Can you work these out from the model? Positions are in its coordinate system, mm. A direction names the side the tool comes from. Coordinates: 2 decimals unless noted, no trailing zeros. Order: outer loops, then holes, each group sorted by start corner. A loop starts at its lowest first (then second) coordinate and runs counter-clockwise, first axis right, second up. Notation, with made-up numbers: M 85.25,-39 L 95.25,-39 A11 cw 95.25,-26 Z; hole C 44.5,-16 d3. An arc over 180 degrees is marked long. Answer as a JSON object with one key per item and string values.
from build123d import *

# Parameters (mm, degrees)
SKETCH1_W                     = 100
SKETCH1_H                     = 100
BOSS_EXTRUDE1_DEPTH           = 2
SKETCH2_W                     = 100
SKETCH2_H                     = 100
SKETCH2_W_2                   = 96
SKETCH2_H_2                   = 96
BOSS_EXTRUDE2_DEPTH           = 30
CHAMFER1_SIZE                 = 10
M3_CLEARANCE_HOLE1_AT_2_COUNT = 2
M3_CLEARANCE_HOLE1_AT_2_PITCH = 10
M3_CLEARANCE_HOLE1_AT_3_COUNT = 2
M3_CLEARANCE_HOLE1_AT_3_PITCH = 19.235384062
M3_CLEARANCE_HOLE1_AT_4_COUNT = 2
M3_CLEARANCE_HOLE1_AT_4_PITCH = 29.154759474
M3_CLEARANCE_HOLE1_AT_5_COUNT = 2
M3_CLEARANCE_HOLE1_AT_5_PITCH = 38.327535793
M3_CLEARANCE_HOLE1_AT_6_COUNT = 2
M3_CLEARANCE_HOLE1_AT_6_PITCH = 48.259714048
CIRPATTERN1_COUNT             = 4


with BuildPart() as part:
    # Sketch1 → Boss-Extrude1 (new body)
    with BuildSketch(Plane(origin=(0, 0, 0), x_dir=(1, 0, 0), z_dir=(0, 1, 0))):
        Rectangle(SKETCH1_W, SKETCH1_H)
    extrude(amount=BOSS_EXTRUDE1_DEPTH)

    # Sketch2 → Boss-Extrude2 (add)
    with BuildSketch(Plane(origin=(0, 2, 0), x_dir=(1, 0, 0), z_dir=(0, 1, 0))):
        Rectangle(SKETCH2_W, SKETCH2_H)
        Rectangle(SKETCH2_W_2, SKETCH2_H_2, mode=Mode.SUBTRACT)
    extrude(amount=BOSS_EXTRUDE2_DEPTH)

    # Chamfer1
    chamfer1_edges = [part.edges().sort_by_distance(p)[0] for p in [
        (-48, 17, -48),
        (-48, 17, 48),
        (48, 17, 48),
        (48, 17, -48),
        (-50, 16, -50),
        (50, 16, -50),
        (50, 16, 50),
        (-50, 16, 50),
    ]]
    chamfer(chamfer1_edges, length=CHAMFER1_SIZE)

    # Sketch3 → M3 Clearance Hole1 (revolve, cut)
    with BuildSketch(Plane(origin=(-24, 25, -48), x_dir=(0, -1, 0), z_dir=(1, 0, 0))):
        Polygon((0, 0), (0, 6.021463052), (1.7, 5), (1.7, 0), align=None)
    m3_clearance_hole1 = revolve(axis=Axis((-24, 25, -41.65), (0, 0, -1)), mode=Mode.SUBTRACT)

    # M3 Clearance Hole1 at 2: M3 Clearance Hole1 ×2
    with Locations(*[(i * M3_CLEARANCE_HOLE1_AT_2_PITCH, 0, 0) for i in range(1, M3_CLEARANCE_HOLE1_AT_2_COUNT)]):
        add(m3_clearance_hole1, mode=Mode.SUBTRACT)

    # M3 Clearance Hole1 at 3: M3 Clearance Hole1 ×2
    with Locations(*[Vector(0.987762965, -0.155962573, 0) * (i * M3_CLEARANCE_HOLE1_AT_3_PITCH) for i in range(1, M3_CLEARANCE_HOLE1_AT_3_COUNT)]):
        add(m3_clearance_hole1, mode=Mode.SUBTRACT)

    # M3 Clearance Hole1 at 4: M3 Clearance Hole1 ×2
    with Locations(*[Vector(0.994691794, -0.102899151, 0) * (i * M3_CLEARANCE_HOLE1_AT_4_PITCH) for i in range(1, M3_CLEARANCE_HOLE1_AT_4_COUNT)]):
        add(m3_clearance_hole1, mode=Mode.SUBTRACT)

    # M3 Clearance Hole1 at 5: M3 Clearance Hole1 ×2
    with Locations(*[Vector(0.991454296, -0.130454513, 0) * (i * M3_CLEARANCE_HOLE1_AT_5_PITCH) for i in range(1, M3_CLEARANCE_HOLE1_AT_5_COUNT)]):
        add(m3_clearance_hole1, mode=Mode.SUBTRACT)

    # M3 Clearance Hole1 at 6: M3 Clearance Hole1 ×2
    with Locations(*[Vector(0.994618409, -0.103606084, 0) * (i * M3_CLEARANCE_HOLE1_AT_6_PITCH) for i in range(1, M3_CLEARANCE_HOLE1_AT_6_COUNT)]):
        add(m3_clearance_hole1, mode=Mode.SUBTRACT)

    # CirPattern1: M3 Clearance Hole1 ×4 about axis
    cirpattern1_axis = Axis((0, 50, 0), (0, -1, 0))
    for i in range(1, CIRPATTERN1_COUNT):
        add(m3_clearance_hole1.rotate(cirpattern1_axis, i * 360 / CIRPATTERN1_COUNT), mode=Mode.SUBTRACT)

    # CirPattern1 copy 1 sketch → CirPattern1 copy 1 (revolve, cut)
    with BuildSketch(Plane(origin=(48, 25, -14), x_dir=(0, -1, 0), z_dir=(0, 0, 1))):
        Polygon((0, 0), (0, 6.021463052), (1.7, 5), (1.7, 0), align=None)
    revolve(axis=Axis((41.65, 25, -14), (1, 0, 0)), mode=Mode.SUBTRACT)

    # CirPattern1 copy 2 sketch → CirPattern1 copy 2 (revolve, cut)
    with BuildSketch(Plane(origin=(14, 25, 48), x_dir=(0, -1, 0), z_dir=(-1, 0, 0))):
        Polygon((0, 0), (0, 6.021463052), (1.7, 5), (1.7, 0), align=None)
    revolve(axis=Axis((14, 25, 41.65), (0, 0, 1)), mode=Mode.SUBTRACT)

    # CirPattern1 copy 3 sketch → CirPattern1 copy 3 (revolve, cut)
    with BuildSketch(Plane(origin=(-48, 25, 14), x_dir=(0, -1, 0), z_dir=(0, 0, -1))):
        Polygon((0, 0), (0, 6.021463052), (1.7, 5), (1.7, 0), align=None)
    revolve(axis=Axis((-41.65, 25, 14), (-1, 0, 0)), mode=Mode.SUBTRACT)

    # CirPattern1 copy 4 sketch → CirPattern1 copy 4 (revolve, cut)
    with BuildSketch(Plane(origin=(48, 22, -5), x_dir=(0, -1, 0), z_dir=(0, 0, 1))):
        Polygon((0, 0), (0, 6.021463052), (1.7, 5), (1.7, 0), align=None)
    revolve(axis=Axis((41.65, 22, -5), (1, 0, 0)), mode=Mode.SUBTRACT)

    # CirPattern1 copy 5 sketch → CirPattern1 copy 5 (revolve, cut)
    with BuildSketch(Plane(origin=(5, 22, 48), x_dir=(0, -1, 0), z_dir=(-1, 0, 0))):
        Polygon((0, 0), (0, 6.021463052), (1.7, 5), (1.7, 0), align=None)
    revolve(axis=Axis((5, 22, 41.65), (0, 0, 1)), mode=Mode.SUBTRACT)

    # CirPattern1 copy 6 sketch → CirPattern1 copy 6 (revolve, cut)
    with BuildSketch(Plane(origin=(-48, 22, 5), x_dir=(0, -1, 0), z_dir=(0, 0, -1))):
        Polygon((0, 0), (0, 6.021463052), (1.7, 5), (1.7, 0), align=None)
    revolve(axis=Axis((-41.65, 22, 5), (-1, 0, 0)), mode=Mode.SUBTRACT)

    # CirPattern1 copy 7 sketch → CirPattern1 copy 7 (revolve, cut)
    with BuildSketch(Plane(origin=(48, 22, 5), x_dir=(0, -1, 0), z_dir=(0, 0, 1))):
        Polygon((0, 0), (0, 6.021463052), (1.7, 5), (1.7, 0), align=None)
    revolve(axis=Axis((41.65, 22, 5), (1, 0, 0)), mode=Mode.SUBTRACT)

    # CirPattern1 copy 8 sketch → CirPattern1 copy 8 (revolve, cut)
    with BuildSketch(Plane(origin=(-5, 22, 48), x_dir=(0, -1, 0), z_dir=(-1, 0, 0))):
        Polygon((0, 0), (0, 6.021463052), (1.7, 5), (1.7, 0), align=None)
    revolve(axis=Axis((-5, 22, 41.65), (0, 0, 1)), mode=Mode.SUBTRACT)

    # CirPattern1 copy 9 sketch → CirPattern1 copy 9 (revolve, cut)
    with BuildSketch(Plane(origin=(-48, 22, -5), x_dir=(0, -1, 0), z_dir=(0, 0, -1))):
        Polygon((0, 0), (0, 6.021463052), (1.7, 5), (1.7, 0), align=None)
    revolve(axis=Axis((-41.65, 22, -5), (-1, 0, 0)), mode=Mode.SUBTRACT)

    # CirPattern1 copy 10 sketch → CirPattern1 copy 10 (revolve, cut)
    with BuildSketch(Plane(origin=(48, 20, 14), x_dir=(0, -1, 0), z_dir=(0, 0, 1))):
        Polygon((0, 0), (0, 6.021463052), (1.7, 5), (1.7, 0), align=None)
    revolve(axis=Axis((41.65, 20, 14), (1, 0, 0)), mode=Mode.SUBTRACT)

    # CirPattern1 copy 11 sketch → CirPattern1 copy 11 (revolve, cut)
    with BuildSketch(Plane(origin=(-14, 20, 48), x_dir=(0, -1, 0), z_dir=(-1, 0, 0))):
        Polygon((0, 0), (0, 6.021463052), (1.7, 5), (1.7, 0), align=None)
    revolve(axis=Axis((-14, 20, 41.65), (0, 0, 1)), mode=Mode.SUBTRACT)

    # CirPattern1 copy 12 sketch → CirPattern1 copy 12 (revolve, cut)
    with BuildSketch(Plane(origin=(-48, 20, -14), x_dir=(0, -1, 0), z_dir=(0, 0, -1))):
        Polygon((0, 0), (0, 6.021463052), (1.7, 5), (1.7, 0), align=None)
    revolve(axis=Axis((-41.65, 20, -14), (-1, 0, 0)), mode=Mode.SUBTRACT)

    # CirPattern1 copy 13 sketch → CirPattern1 copy 13 (revolve, cut)
    with BuildSketch(Plane(origin=(48, 20, 24), x_dir=(0, -1, 0), z_dir=(0, 0, 1))):
        Polygon((0, 0), (0, 6.021463052), (1.7, 5), (1.7, 0), align=None)
    revolve(axis=Axis((41.65, 20, 24), (1, 0, 0)), mode=Mode.SUBTRACT)

    # CirPattern1 copy 14 sketch → CirPattern1 copy 14 (revolve, cut)
    with BuildSketch(Plane(origin=(-24, 20, 48), x_dir=(0, -1, 0), z_dir=(-1, 0, 0))):
        Polygon((0, 0), (0, 6.021463052), (1.7, 5), (1.7, 0), align=None)
    revolve(axis=Axis((-24, 20, 41.65), (0, 0, 1)), mode=Mode.SUBTRACT)

    # CirPattern1 copy 15 sketch → CirPattern1 copy 15 (revolve, cut)
    with BuildSketch(Plane(origin=(-48, 20, -24), x_dir=(0, -1, 0), z_dir=(0, 0, -1))):
        Polygon((0, 0), (0, 6.021463052), (1.7, 5), (1.7, 0), align=None)
    revolve(axis=Axis((-41.65, 20, -24), (-1, 0, 0)), mode=Mode.SUBTRACT)


solid = part.part
Item 1: I want a section at B-B, the plane x = 24. Write out the boundary of the cut face in (y, z).
Answers follow:
{"outline": "M 0,-50 L 18.3,-50 L 18.3,-48 L 2,-48 L 2,48 L 23.3,48 L 23.3,50 L 0,50 Z; M 21.7,-50 L 32,-50 L 32,-48 L 21.7,-48 Z; M 26.7,48 L 32,48 L 32,50 L 26.7,50 Z"}
Item 2: If we mould it in two halves opening along Y, with no side actions, what happens to faces 6 (the cylindrical face through (4.49, 20.38, -48.99)), 7 (the flat face through (-1, 0, -1)), 8 (the flat face through (-43, 17, -43)), 9 (the flat face through (-18.8, 32, -48.4))? For each: pulls with the +Y half, pulls with the -Y half, needs draft (parallel to the pull), parting line crosses it, or undercut.
Answers follow:
{"face 6": "undercut", "face 7": "pulls with the -Y half", "face 8": "needs draft", "face 9": "pulls with the +Y half"}
Item 3: I want a section at A-A, the plane z = -5. Write out the boundary of the cut face in (x, y).
Answers follow:
{"outline": "M -50,0 L 50,0 L 50,20.3 L 48,20.3 L 48,2 L -48,2 L -48,20.3 L -50,20.3 Z; M -50,23.7 L -48,23.7 L -48,32 L -50,32 Z; M 48,23.7 L 50,23.7 L 50,32 L 48,32 Z"}
Item 4: I want a section at D-D, the plane x = -17. Write out the boundary of the cut face in (y, z), plus the area to 3 significant figures.
Answers follow:
{"outline": "M 0,-50 L 32,-50 L 32,-48 L 2,-48 L 2,48 L 32,48 L 32,50 L 0,50 Z", "area": "320 mm^2"}
Item 5: I'm going to push flat-ended pins straight in: pin 1 (5 mm diameter, centred on x = 30.5, z = 6, fed in from +Y); pin 2 (3 mm diameter, centred on y = 22, z = 5, fed in from +X); pin 3 (3 mm diameter, centred on x = -24, y = 25, fed in from -Z); pin 4 (3 mm diameter, centred on x = -14, y = 20, fed in from +Z). Where does each tip first touch, or does it pass through?
Answers follow:
{"pin 1": "stops at y = 2", "pin 2": "passes through", "pin 3": "stops at z = 48", "pin 4": "stops at z = -48"}
Item 6: Please list where these lines run through material, in increasing order: line 1 (Z direction, x = 35, y = 2.5); line 2 (Z direction, x = 49.2, y = 20).
Answers follow:
{"line 1": "z = -50 to -48, 48 to 50", "line 2": "z = -40.8 to 12.3, 15.7 to 22.3, 25.7 to 40.8"}
Item 7: Which directions (+Z, -Z, +X, -X, +Y, -Y) give clear straight access to the entire face, cutting with the end or side of a thin tool? Please do faces 1 (the cylindrical face through (-24.51, 23.38, -48.99)), 2 (the flat face through (-1, 2, -1)), 3 (the cylindrical face through (-13.49, 18.38, 48.99)), 4 (the cylindrical face through (-48.99, 18.38, -23.49)), 5 (the flat face through (-50, 16, 1)).
Answers follow:
{"face 1": "-Z", "face 2": "+Y", "face 3": "+Z", "face 4": "-X", "face 5": "+Z, -Z, -X, +Y, -Y"}
Item 8: I want a section at C-C, the plane y = 10. Write out the boundary of the cut face in (x, z), plus the area to 3 significant figures.
Answers follow:
{"outline": "M -50,-40 L -40,-50 L 40,-50 L 50,-40 L 50,40 L 40,50 L -40,50 L -50,40 Z; hole M -48,-38 L -38,-48 L 38,-48 L 48,-38 L 48,38 L 38,48 L -38,48 L -48,38 Z", "area": "784 mm^2"}
